Check sheet for the modelled part. Datum: model origin and axes. Units: mm. Coordinates: 2 decimals unless noted, no trailing zeros. Order: outer loops, then holes, each group sorted by start corner. A loop starts at its lowest first (then second) coordinate and runs counter-clockwise, first axis right, second up. Notation, with made-up numbers: (63.25, 26) -> (86.25, 26) arc R16 ccw to (86.25, 56) -> close; hole circle Ø4 at (-28, 6.5). An arc over 180 degrees is marked (long way). Put each result on its own line as item: value. Start each with the question number.
```python
from build123d import *

# Parameters (mm, degrees)
F0_W      = 30
F0_H      = 30
F1_DEPTH  = 15
F5_R      = 2
F6_DEPTH  = 1.5
F7_R      = 2
F8_DEPTH  = 1.5
F9_R      = 2
F10_DEPTH = 1.5
F11_R     = 2
F12_DEPTH = 1.5
F13_R     = 2
F14_DEPTH = 1.5
F15_R     = 2
F16_DEPTH = 1.5


with BuildPart() as f1:
    # F0 (on Top) → F1 (new body, symmetric)
    with BuildSketch(Plane.XY):
        Rectangle(F0_W, F0_H)
    extrude(amount=F1_DEPTH, both=True)


with BuildPart() as f3:
    # F2 (on Top) → F3 (revolve)
    with BuildSketch(Plane.XY):
        with BuildLine():
            ThreePointArc((0, -20), (20, 0), (0, 20))
            Line((0, 20), (0, -20))
        make_face()
    revolve(axis=Axis((0, 0, 0), (0, -1, 0)))


with BuildPart() as f1_1:
    add(f1.part)

    # F4: intersect F3
    add(f3.part, mode=Mode.INTERSECT)

    # F5 (on face) → F6 (cut)
    with BuildSketch(Plane(origin=(0, 0, -15), x_dir=(1, 0, 0), z_dir=(0, 0, -1))):
        Circle(F5_R)
    extrude(amount=-F6_DEPTH, mode=Mode.SUBTRACT)

    # F7 (on face) → F8 (cut)
    with BuildSketch(Plane.XY.offset(15)):
        with Locations((0, 5)):
            Circle(F7_R)
        with Locations((6.5, 5)):
            Circle(F7_R)
        with Locations((0, -5)):
            Circle(F7_R)
        with Locations((6.5, -5)):
            Circle(F7_R)
        with Locations((-6.5, -5)):
            Circle(F7_R)
        with Locations((-6.5, 5)):
            Circle(F7_R)
    extrude(amount=-F8_DEPTH, mode=Mode.SUBTRACT)

    # F9 (on face) → F10 (cut)
    with BuildSketch(Plane(origin=(-15, 0, 0), x_dir=(0, -1, 0), z_dir=(-1, 0, 0))):
        with Locations((5.303301, 5.303301)):
            Circle(F9_R)
        with Locations((-5.303301, -5.303301)):
            Circle(F9_R)
    extrude(amount=-F10_DEPTH, mode=Mode.SUBTRACT)

    # F11 (on face) → F12 (cut)
    with BuildSketch(Plane.YZ.offset(15)):
        with Locations((5.303301, 5.303301)):
            Circle(F11_R)
        Circle(F11_R)
        with Locations((-5.303301, 5.303301)):
            Circle(F11_R)
        with Locations((5.303301, -5.303301)):
            Circle(F11_R)
        with Locations((-5.303301, -5.303301)):
            Circle(F11_R)
    extrude(amount=-F12_DEPTH, mode=Mode.SUBTRACT)

    # F13 (on face) → F14 (cut)
    with BuildSketch(Plane.XZ.offset(15)):
        with Locations((5.303301, 5.303301)):
            Circle(F13_R)
        Circle(F13_R)
        with Locations((-5.303301, -5.303301)):
            Circle(F13_R)
    extrude(amount=-F14_DEPTH, mode=Mode.SUBTRACT)

    # F15 (on face) → F16 (cut)
    with BuildSketch(Plane(origin=(0, 15, 0), x_dir=(-1, 0, 0), z_dir=(0, 1, 0))):
        with Locations((5.303301, 5.303301)):
            Circle(F15_R)
        with Locations((-5.303301, 5.303301)):
            Circle(F15_R)
        with Locations((5.303301, -5.303301)):
            Circle(F15_R)
        with Locations((-5.303301, -5.303301)):
            Circle(F15_R)
    extrude(amount=-F16_DEPTH, mode=Mode.SUBTRACT)


solid = f1_1.part
```
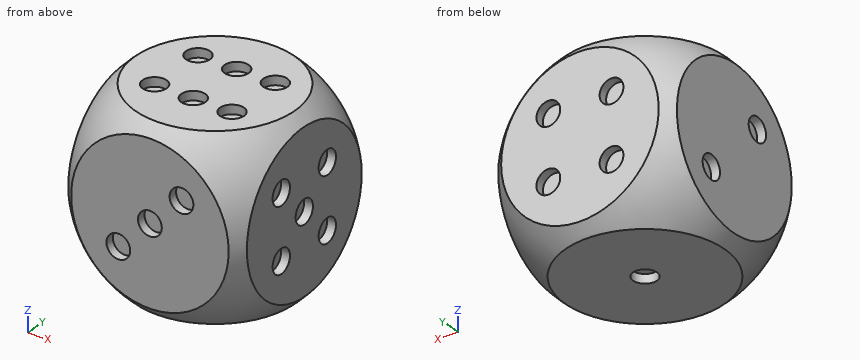
1) Sectioned sample at A-A (x = 0). Record the boundary of the cut face in (y, z), plus the area to 3 significant figures.
2) Gauge pin test, flat ends, axial feed: pin 1 (2 mm diameter, centred on x = -5, z = -6, fed in from -Y); pin 2 (3.5 mm diameter, centred on x = -5.3, z = -5.3, fed in from +Y). Record the tip position at first contact, or that the pin passes through.
3) Sectioned sample at D-D (x = -9.25). Record the boundary of the cut face in (y, z), plus the area to 3 significant figures.
4) Scan lines: line 1 along Y through (x, z) = (6.5, 14.3); line 2 along Z through (x, y) = (-1, 6); line 3 along Z through (x, y) = (14.15, 0). Record each from-to range of solid material in increasing order. Write a range as [from, to].
5) Sectioned sample at B-B (z = 0). Record the boundary of the cut face in (x, y), plus the area to 3 significant figures.
Entries:
1. outline: (-15, -13.23) arc R20 ccw to (-13.23, -15) -> (-2, -15) -> (-2, -13.5) -> (2, -13.5) -> (2, -15) -> (13.23, -15) arc R20 ccw to (15, -13.23) -> (15, 13.23) arc R20 ccw to (13.23, 15) -> (7, 15) -> (7, 13.5) -> (3, 13.5) -> (3, 15) -> (-3, 15) -> (-3, 13.5) -> (-7, 13.5) -> (-7, 15) -> (-13.23, 15) arc R20 ccw to (-15, 13.23) -> (-15, 2) -> (-13.5, 2) -> (-13.5, -2) -> (-15, -2) -> close
1. area: 870 mm2
2. pin 1: stops at y = -13.5
2. pin 2: stops at y = 13.5
3. outline: (-15, -9.46) arc R17.73 ccw to (-9.46, -15) -> (9.46, -15) arc R17.73 ccw to (15, -9.46) -> (15, 9.46) arc R17.73 ccw to (9.46, 15) -> (-9.46, 15) arc R17.73 ccw to (-15, 9.46) -> close
3. area: 848 mm2
4. line 1: y = [-12.38, -7], [-3, 3], [7, 12.38]
4. line 2: z = [-15, 13.5]
4. line 3: z = [-14.13, -2], [2, 14.13]
5. outline: (-15, -13.23) arc R20 ccw to (-13.23, -15) -> (-2, -15) -> (-2, -13.5) -> (2, -13.5) -> (2, -15) -> (13.23, -15) arc R20 ccw to (15, -13.23) -> (15, -2) -> (13.5, -2) -> (13.5, 2) -> (15, 2) -> (15, 13.23) arc R20 ccw to (13.23, 15) -> (-13.23, 15) arc R20 ccw to (-15, 13.23) -> close
5. area: 882 mm2
